Input: part model. Units: mm. Frame: model coordinates. A direction names the side the tool comes from. Give positions to 0.01 mm unless a question says otherwise; leave off trailing zeros. Order: outer loops, then holes, each group sorted by start corner. A loop starts at its lowest first (then second) coordinate and runs counter-clockwise, first axis right, second up. Notation, with made-up numbers: M 8,-17 L 39,-17 A27 ccw 39,18 Z; hole C 11,-7 d6. An arc over 180 degrees is marked long. Use a Markdown table: item, result.
Autodesk Inventor part; units mm, degrees
ref_plane "Work Plane1" through (13.9848, 0, 0) normal (0, 0, 1) x (-1, 0, 0)
ref_plane "YZ Plane" through (0, 0, 0) normal (1, 0, 0) x (0, 1, 0)
ref_plane "XZ Plane" through (0, 0, 0) normal (0, 1, 0) x (-1, 0, 0)
sketch "Sketch1" plane through (0, 0, 0) normal (1, 0, 0) x (0, 1, 0)
  line L0 (2.3094, -4) -> (-2.3094, -4)
  line L1 (-2.3094, -4) -> (-4.6188, 0)
  line L2 (-4.6188, 0) -> (-2.3094, 4)
  line L3 (-2.3094, 4) -> (2.3094, 4)
  line L4 (2.3094, 4) -> (4.6188, 0)
  line L5 (4.6188, 0) -> (2.3094, -4)
  point P0 (0, 0)
  point P1 (0, 0)
  dimension "d0" = 9.2376
extrude "Body" add sketch "Sketch1" along normal blind 4.4
sketch "Sketch2" plane through (4.4, 0, 0) normal (1, 0, 0) x (0, 0, -1)
  circle A0 centre (0, 0) radius 4
  dimension "d7" = 8
extrude "Ring" add sketch "Sketch2" along normal blind 2.4
sketch "Sketch3" plane through (0, 0, 0) normal (0, 0, 1) x (1, 0, 0)
  line L0 (0, 2.3094) -> (0, 4.6188)
  line L1 (0, 4.6188) -> (4.4, 4.6188)
  line L2 (4.4, 2.3094) -> (4.4, 4.6188)
  line L3 (-0.88, 0) -> (5.28, 0)
  line L4 (0, 4) -> (0.3573, 4.6188)
  line L5 (4.0427, 4.6188) -> (4.4, 4)
  dimension "d3" = 30
  dimension "d4" = 30
  dimension "d5" = 8
  dimension "d6" = 8
revolve "Chamfer1" cut sketch "Sketch3" angle 360 about axis through (-10, 0, 0) along (1, 0, 0)
sketch "Sketch4" plane through (0, 0, 0) normal (-1, 0, 0) x (0, 0, 1)
  line L0 (0, -6.4663) -> (0, 6.4663)
  line L1 (-5.6, 0) -> (5.6, 0)
  point P0 (0, 0)
hole "Thread" at (0, 0, 0) direction (1, 0, 0) diameter 4.134 end through all
chamfer "Chamfer2" distance 0.433 angle 30 1 edges at (0, 0, -2.067) measured on face at (0, -3.336, 0.083)
chamfer "Chamfer3" distance 0.433 angle 30 1 edges at (6.8, 0, -2.067) measured on face at (6.8, -0.484, -3.2969)
ref_plane "Work Plane1" through (13.9848, 0, 0) normal (0, 0, 1) x (-1, 0, 0)
equation "\"d0\" = 1.1547 * SW"
equation "\"d1\" = KOH1"
equation "\"d7\" = SD2"
equation "\"d8\" = KOH - KOH1"
equation "\"d3\" = ANG1"
equation "\"d4\" = ANG2"
equation "\"d5\" = SW0"
equation "\"d6\" = SW01"
equation "\"d10\" = -0.5 * GD1 + 0.5 * NND"
equation "\"d46\" = -0.5 * GD1 + 0.5 * NND"
equation "\"d12\" = -0.5 * GD1 + 0.5 * NND"
equation "\"d47\" = -0.5 * GD1 + 0.5 * NND"
equation "\"ANG1\" = 30deg"
equation "\"ANG2\" = 30deg"
equation "\"NND\" = 5"
equation "\"KOH1\" = 4.4"
equation "\"KOH\" = 6.8"
equation "\"SW\" = 8"
equation "\"SW0\" = SW"
equation "\"SW01\" = SW"
equation "\"SD2\" = SW"
equation "\"GUL\" = 0.541266 * PTC"
equation "\"THREADDIA\" = 5"
equation "\"TOA\" = 30deg"
equation "\"PTC\" = 0.8"
equation "\"E0\" = 1.155 * SW"
equation "\"GAL\" = 0.541266 * PTC"
properties part number "SS-ISO 7040 - M5" material "Steel, Mild"
1) Reachability of faces 1 (the face through (5.583, 3.905, 0.867)), 2 (the face through (2, 0, -4)) from +Z, -Z, +X, -X, +Y, -Y: full face, straight path, thin tool, end or side. Return the list, or none.
Response values:
| item | result |
|---|---|
| face 1 | +X |
| face 2 | -Z, +X, -X, +Y, -Y |
2) Material intervals for line 1 (Z direction, x = 4.5, y = 0); line 2 (Y direction, x = 6.75, z = 1.5), sorted ascending. Write a range as from..to.
Response values:
| item | result |
|---|---|
| line 1 | z = -4..-2.07, 2.07..4 |
| line 2 | y = -3.71..-1.89, 1.89..3.71 |
3) Cut plane A-A on x = 1.5. Return loops of the section in (y, z).
Response values:
| item | result |
|---|---|
| outline | M -4.62,0 L -2.31,-4 L 2.31,-4 L 4.62,0 L 2.31,4 L -2.31,4 Z; hole C 0,0 d4.13 |
4) First-contact query: pin 1 Ø3.5 at (y, z) = (0, 0) entering from -X; pin 2 Ø2 at (x, z) = (4, 3) entering from +Y. Flat tips, straight axial feed; report the tip coordinate or a pass-through.
Response values:
| item | result |
|---|---|
| pin 1 | passes through |
| pin 2 | stops at y = 3.46 |
5) Cut plane B-B on x = 6. Return loops of the section in (y, z), and give its area (3 significant figures).
Response values:
| item | result |
|---|---|
| outline | C 0,0 d8; hole C 0,0 d4.13 |
| area | 36.8 mm² |
